Could you check a few things on this drawing? It's one solid part, dimensions in mm from its lowest x, y, z. A direction names the side the tool comes from. Coordinates: 2 decimals unless noted, no trailing zeros. Write each loop counter-clockwise with the first axis right and the second up, starting at its lowest first coordinate (ties: lowest second). Pieces come first, ordered by that corner, then holes. Notation, with made-up numbers: (-11, -39.75) - (35, -39.75) arc R22 cw to (35, -26.75) - close; hole circle Ø9 at (72, 73). An arc over 180 degrees is marked (long way). Answer as a JSON object with one key per item and string values. Group by question number.
1) Will these pins go through, and if not, where does the flat tip stop? pin 1 Ø12 at (x, z) = (10, 25) entering from -Y; pin 2 Ø5 at (y, z) = (32.5, 51) entering from +X; pin 3 Ø5 at (x, y) = (10, 6.5) entering from -Z.
2) If we section it at B-B (y = 27.5): Write out the boundary of the cut face in (x, z), plus the area to 3 significant figures.
3) If we section it at D-D (z = 60.5): Write out the boundary of the cut face in (x, y).
4) On a 3-axis mill with a long thin cutter (end or side, diameter ignored), from which of +Z, -Z, +X, -X, +Y, -Y can I reach the whole of each face in a straight line? I mean the marked faces 1, 2 and 3. Say none if no direction works.
5) Please list where these lines run through material, in increasing order: line 1 along Y through (x, z) = (43.5, 40); line 2 along Z through (x, y) = (43, 6); line 3 along X through (y, z) = (43, 37) (1 decimal).
6) If we section it at A-A (x = 41.5): Write out the boundary of the cut face in (y, z) (1 decimal), plus the area to 3 significant figures.
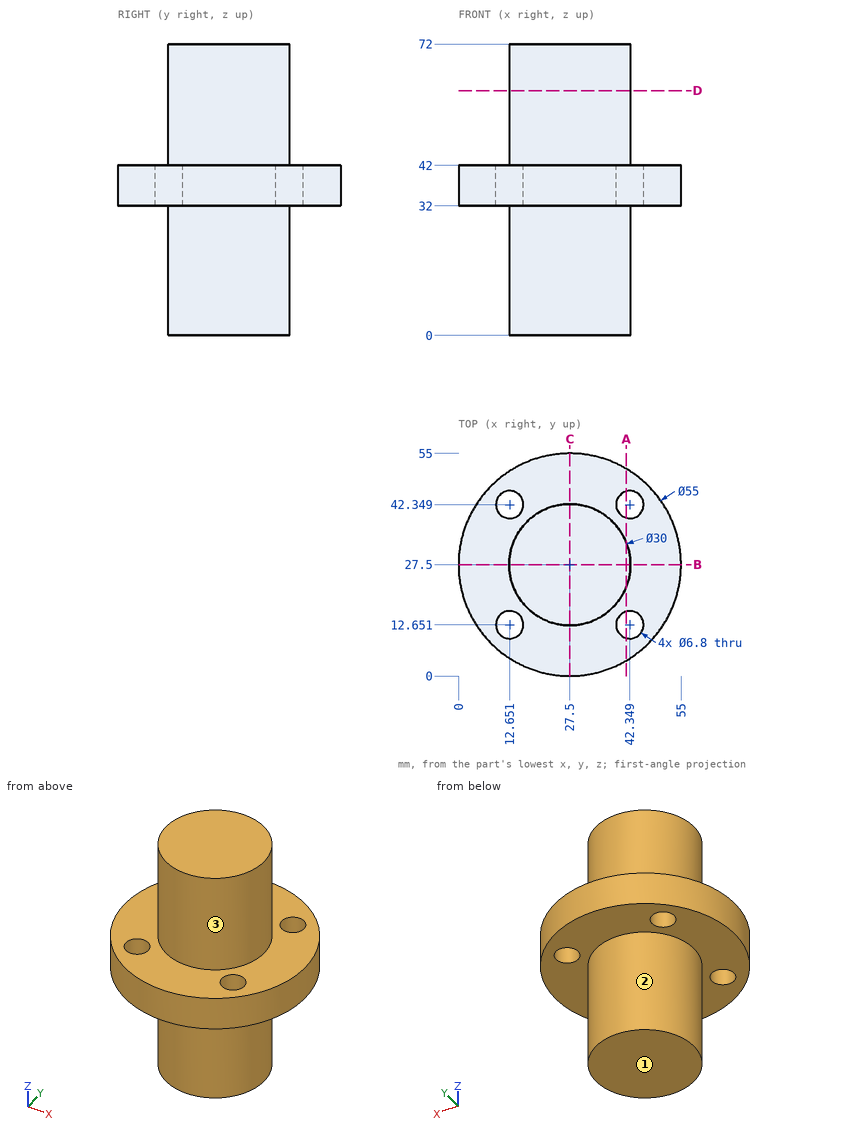
Here are the results:
{
 "1": {"pin 1": "stops at y = 17.87", "pin 2": "stops at x = 42.29", "pin 3": "stops at z = 32"},
 "2": {"outline": "(0, 32) - (12.5, 32) - (12.5, 0) - (42.5, 0) - (42.5, 32) - (55, 32) - (55, 42) - (42.5, 42) - (42.5, 72) - (12.5, 72) - (12.5, 42) - (0, 42) - close", "area": "2,410 mm²"},
 "3": {"outline": "circle Ø30 at (27.5, 27.5)"},
 "4": {"face 1": "-Z, +X, -X, +Y, -Y", "face 2": "-Z", "face 3": "+Z"},
 "5": {"line 1": "y = 5.13 to 9.45, 15.85 to 39.15, 45.55 to 49.87", "line 2": "z = 32 to 42", "line 3": "x = 4.8 to 9.3, 16 to 39, 45.7 to 50.2"},
 "6": {"outline": "(3.8, 32) - (9.4, 32) - (9.4, 42) - (3.8, 42) - close; (15.9, 32) - (22.1, 32) - (22.1, 0) - (32.9, 0) - (32.9, 32) - (39.1, 32) - (39.1, 42) - (32.9, 42) - (32.9, 72) - (22.1, 72) - (22.1, 42) - (15.9, 42) - close; (45.6, 32) - (51.2, 32) - (51.2, 42) - (45.6, 42) - close", "area": "1,010 mm²"}
}
